```python
from build123d import *

# Parameters (mm, degrees)
F0_W         = 7.9375
F0_H         = 7.9375
F0_R         = 2.54
F1_DEPTH     = 7.9375
F2_R         = 3.46075
F2_R_2       = 2.54
F3_DEPTH     = 7.9375
F4_T3_DEPTH  = 27.78125
F4_S4_R      = 3.46075
F4_T5_DEPTH  = 16
F4_T8_DEPTH  = 27.78125
F4_S9_R      = 3.46075
F4_T10_DEPTH = 16
F4_T13_DEPTH = 27.78125
F4_T16_DEPTH = 27.78125


# Not quite as in the source:
# - a fillet or chamfer that OpenCascade refuses, or shapes differently, is made with other operations: its cross-section is extruded or revolved along the edge and cut away or added


with BuildPart() as f1:
    # F0 (on Top) → F1 (new body)
    with BuildSketch(Plane.XY):
        Rectangle(F0_W, F0_H)
        Circle(F0_R, mode=Mode.SUBTRACT)
    extrude(amount=F1_DEPTH)

    # F2 (on face) → F3 (join)
    with BuildSketch(Plane(origin=(0, 3.96875, 0), x_dir=(-1, 0, 0), z_dir=(0, 1, 0))):
        with Locations((0, 3.96875)):
            Circle(F2_R)
        with Locations((0, 3.96875)):
            Circle(F2_R_2, mode=Mode.SUBTRACT)
    extrude(amount=F3_DEPTH)

    # F4: fillet of radius 3.96875 on 4 edges, made by hand


with BuildPart() as f4_tool1:
    # F4_s2 → F4_t3 (new body)
    with BuildSketch(Plane.XY.offset(-9.921875)):
        with BuildLine():
            ThreePointArc((0, 3.96875), (-2.8063300378, 2.8063300378), (-3.96875, 0))
            Line((-3.96875, 0), (-3.96875, 3.96875))
            Line((-3.96875, 3.96875), (0, 3.96875))
        make_face()
    extrude(amount=F4_T3_DEPTH)

    # F4_s4 → F4_t5 (cut, symmetric)
    with BuildSketch(Plane.XZ.offset(-2)):
        with Locations((0, 3.96875)):
            Circle(F4_S4_R)
    extrude(amount=F4_T5_DEPTH, both=True, mode=Mode.SUBTRACT)


with BuildPart() as f4_tool6:
    # F4_s7 → F4_t8 (new body)
    with BuildSketch(Plane.XY.offset(-9.921875)):
        with BuildLine():
            ThreePointArc((3.96875, 0), (2.8063300378, 2.8063300378), (0, 3.96875))
            Line((0, 3.96875), (3.96875, 3.96875))
            Line((3.96875, 3.96875), (3.96875, 0))
        make_face()
    extrude(amount=F4_T8_DEPTH)

    # F4_s9 → F4_t10 (cut, symmetric)
    with BuildSketch(Plane.XZ.offset(-2)):
        with Locations((0, 3.96875)):
            Circle(F4_S9_R)
    extrude(amount=F4_T10_DEPTH, both=True, mode=Mode.SUBTRACT)


with BuildPart() as f4_tool11:
    # F4_s12 → F4_t13 (new body)
    with BuildSketch(Plane.XY.offset(-9.921875)):
        with BuildLine():
            ThreePointArc((3.96875, 0), (2.8063300378, -2.8063300378), (0, -3.96875))
            Line((0, -3.96875), (3.96875, -3.96875))
            Line((3.96875, -3.96875), (3.96875, 0))
        make_face()
    extrude(amount=F4_T13_DEPTH)


with BuildPart() as f4_tool14:
    # F4_s15 → F4_t16 (new body)
    with BuildSketch(Plane.XY.offset(-9.921875)):
        with BuildLine():
            ThreePointArc((0, -3.96875), (-2.8063300378, -2.8063300378), (-3.96875, 0))
            Line((-3.96875, 0), (-3.96875, -3.96875))
            Line((-3.96875, -3.96875), (0, -3.96875))
        make_face()
    extrude(amount=F4_T16_DEPTH)


with BuildPart() as f1_1:
    add(f1.part)

    # F4_t17: cut F4_tool1, F4_tool6, F4_tool11, F4_tool14
    add([f4_tool1.part, f4_tool6.part, f4_tool11.part, f4_tool14.part], mode=Mode.SUBTRACT)


solid = f1_1.part
```
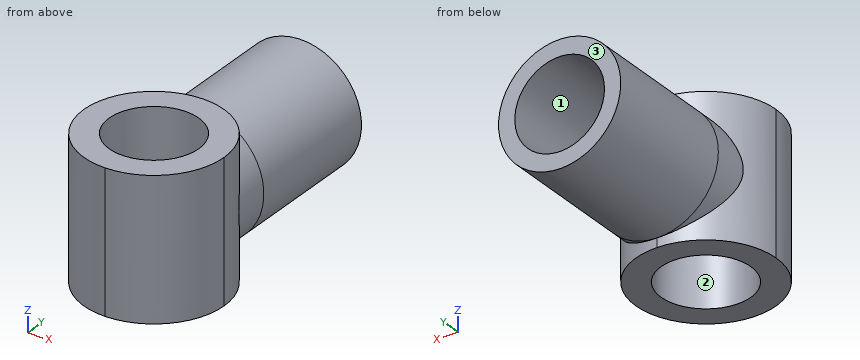
Input: part model. Units: mm. Frame: model coordinates. Face numbers are marked on the shaded views. Round coordinates to 2 decimals unless told otherwise and drop trailing zeros. Order: outer loops, then holes, each group sorted by start corner. A loop starts at its lowest first (then second) coordinate and runs counter-clockwise, first axis right, second up. Notation, with made-up numbers: (-37, 14) - (6, 14) arc R32 cw to (6, 45) - close; hole circle Ø3 at (-18.5, 21.25). An arc over 180 degrees is marked (long way). One line per question, with ' | ' between items. Start each with the question number.
1) Pull-direction query (Y, two-part tool) for the marked faces 1, 2 and 3; classes: +Y half, -Y half, draft (parallel to the pull), parting line (faces both ways), or undercut.
2) Cut plane B-B, the plane y = -1.25. Return the cut outline in (x, z).
3) Contact query for flat-ended pins moving along their axis: P1, Ø1.5, axis at x = 1, z = 4, coming from the +Y side; P2, Ø3, axis at y = 6, z = 4.5, coming from the +X side; P3, Ø3, axis at y = 7.5, z = 2, coming from the +X side; P4, Ø4.5, axis at x = 0, y = 0, coming from the -Z side. Output: stop coordinate, or through.
4) Cut plane A-A, the plane x = 1. Return the cut outline in (y, z).
5) Ray query, probe 1 along Y at (x, z) = (0, 3.25); probe 2 along Z at (x, y) = (0, 10); probe 3 along X at (y, z) = (9, 4). Return the intervals inside material, ascending.
6) Cut plane C-C, the plane z = 4.75. Return the cut outline in (x, y), then the cut area to 3 significant figures.
7) Cut plane D-D, the plane x = -2. Return the cut outline in (y, z), then the cut area to 3 significant figures.
Worked out:
1) face 1: draft | face 2: undercut | face 3: +Y half
2) outline: (-3.77, 0) - (-2.21, 0) - (-2.21, 7.94) - (-3.77, 7.94) - close; (2.21, 0) - (3.77, 0) - (3.77, 7.94) - (2.21, 7.94) - close
3) P1: stops at y = 3.97 | P2: stops at x = 3.46 | P3: stops at x = 3.43 | P4: passes through
4) outline: (-3.84, 0) - (-2.33, 0) - (-2.33, 7.94) - (-3.84, 7.94) - close; (2.33, 0) - (3.84, 0) - (3.84, 0.66) - (11.91, 0.66) - (11.91, 1.63) - (3.97, 1.63) - (3.97, 6.3) - (11.91, 6.3) - (11.91, 7.28) - (3.84, 7.28) - (3.84, 7.94) - (2.33, 7.94) - close
5) probe 1: y = -3.97 to -2.54, 2.54 to 3.97 | probe 2: z = 0.51 to 1.43, 6.51 to 7.43 | probe 3: x = -3.46 to -2.54, 2.54 to 3.46
6) outline: (-3.37, 2.09) arc R3.97 ccw (long way) to (3.37, 2.09) - (3.37, 11.91) - (2.42, 11.91) - (2.42, 3.97) - (-2.42, 3.97) - (-2.42, 11.91) - (-3.37, 11.91) - close; hole circle Ø5.08 at (0, 0) | area: 48.1 mm^2
7) outline: (-3.43, 0) - (-1.57, 0) - (-1.57, 7.94) - (-3.43, 7.94) - close; (1.57, 0) - (3.43, 0) - (3.43, 1.14) - (11.91, 1.14) - (11.91, 2.4) - (3.97, 2.4) - (3.97, 5.53) - (11.91, 5.53) - (11.91, 6.79) - (3.43, 6.79) - (3.43, 7.94) - (1.57, 7.94) - close | area: 52.6 mm^2
